Check sheet for the modelled part. Datum: model origin and axes. Units: mm. Face numbers are marked on the shaded views. A direction names the side the tool comes from. Give positions to 0.01 mm unless a question says otherwise; leave off trailing zeros. Loops run counter-clockwise (first coordinate to the right, second up) from the corner with the lowest first, then second, coordinate; pieces in that order, holes last. Notation, with made-up numbers: (83, -34.75) - (142, -34.75) arc R13 cw to (142, -16.75) - close; hole circle Ø7 at (80.25, 26). An arc over 180 degrees is marked (long way). Answer in a Markdown table with one row per item. Add a question column.
(1) Draft check along X on the marked faces 4, 5 and 6. Enter one of: released by +X, released by -X, zero draft, split by the parting line, or undercut.
(2) Set-up check for the marked faces 1, 2 and 3: record each of +Z, -Z, +X, -X, +Y, -Y from which the full face is reachable in a straight line by a thin tool's end or side.
(3) Thickness scan on L1, parallel to Z at x = -60, y = -1; L2, parallel to Z at x = -29, y = -3.5; L3, parallel to X at y = -0.5, z = -1.5. Record the ranges inside material, lowest first.
(4) Sectioned sample at C-C on y = -4.25. Enter the section's corners in (x, z) (1 decimal).
(5) Sectioned sample at D-D on x = -14. Enter the section's corners in (y, z), then the cut area to 3 significant figures.
(6) Sectioned sample at A-A on y = -11.5. Enter the section's corners in (x, z), then the cut area to 3 significant figures.
(7) Go/stop test with flat-tipped pins: P1, Ø13, axis at x = -14, z = 34.5, coming from the +Y side; P2, Ø1, axis at x = -86, z = 30, coming from the -Y side; P3, Ø4, axis at y = -6, z = 29, coming from the -X side. Record where each tip stops, or that it passes through.
(8) Sectioned sample at B-B on x = -56.5. Enter the section's corners in (y, z), then the cut area to 3 significant figures.
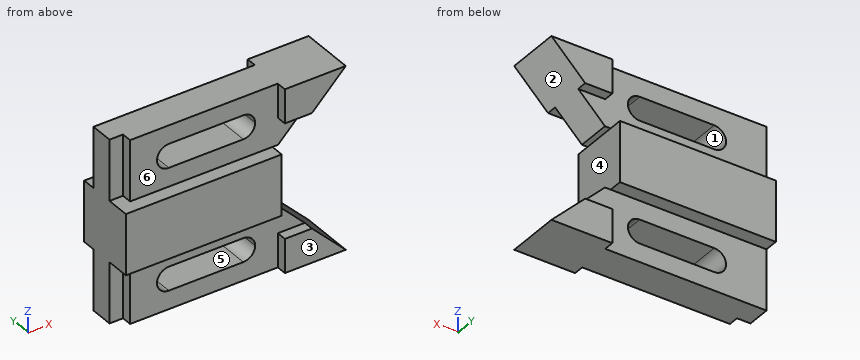
from build123d import *

# Parameters (mm, degrees)
F1_DEPTH = 104.648
F2_W     = 75.946
F2_H     = 4.826
F2_W_2   = 6.35
F3_DEPTH = 28.575
F5_DEPTH = 22.099
F7_DEPTH = 26.925
F9_DEPTH = 28.449


# Not quite as in the source:
# - a pattern or mirror of a feature is missing from the dataset's text; its kind, count and spacing are read off the source's solid


with BuildPart() as f1:
    # F0 (on Right) → F1 (new body)
    with BuildSketch(Plane.YZ):
        Polygon((7.874, -14.2875), (14.224, -14.2875), (14.224, 14.2875), (7.874, 14.2875), (-7.874, 14.2875), (-14.224, 14.2875), (-14.224, -14.2875), (-7.874, -14.2875), align=None)
        Polygon((-7.874, 14.2875), (7.874, 14.2875), (7.874, 26.924), (12.7, 26.924), (12.7, 42.8625), (0, 42.8625), (-12.7, 42.8625), (-12.7, 26.924), (-7.874, 26.924), align=None)
        Polygon((7.874, -26.924), (7.874, -14.2875), (-7.874, -14.2875), (-7.874, -26.924), (-12.7, -26.924), (-12.7, -42.8625), (0, -42.8625), (12.7, -42.8625), (12.7, -26.924), align=None)
    extrude(amount=-F1_DEPTH)

    # F2 (on face) → F3 (cut)
    with BuildSketch(Plane.XY.offset(42.8625)):
        Polygon((-98.298, -7.874), (-104.648, -7.874), (-104.648, -12.7), (-28.702, -12.7), (-28.702, -7.874), align=None)
        with Locations((-66.675, 10.287)):
            Rectangle(F2_W, F2_H)
        with Locations((-101.473, -5.461)):
            Rectangle(F2_W_2, F2_H)
    f3 = extrude(amount=-F3_DEPTH, mode=Mode.SUBTRACT)

    # F3_copies: F3 across plane
    add(f3.mirror(Plane(origin=(0, 0, 0), x_dir=(-1, 0, 0), z_dir=(0, 0, -1))), mode=Mode.SUBTRACT)

    # F4 (on face) → F5 (cut, through all)
    with BuildSketch(Plane.XZ.offset(7.874)):
        with BuildLine():
            ThreePointArc((-80.01, -34.2265), (-76.0586873067, -32.5898126933), (-74.422, -28.6385))
            ThreePointArc((-74.422, -28.6385), (-76.0586873067, -24.6871873067), (-80.01, -23.0505))
            ThreePointArc((-80.01, -23.0505), (-85.598, -28.6385), (-80.01, -34.2265))
        make_face()
        with BuildLine():
            ThreePointArc((-80.01, -23.0505), (-76.0586873067, -24.6871873067), (-74.422, -28.6385))
            ThreePointArc((-74.422, -28.6385), (-76.0586873067, -32.5898126933), (-80.01, -34.2265))
            Line((-80.01, -34.2265), (-44.958, -34.2265))
            ThreePointArc((-44.958, -34.2265), (-50.546, -28.6385), (-44.958, -23.0505))
            Line((-44.958, -23.0505), (-80.01, -23.0505))
        make_face()
        with BuildLine():
            ThreePointArc((-39.37, -28.6385), (-41.0066873067, -24.6871873067), (-44.958, -23.0505))
            ThreePointArc((-44.958, -23.0505), (-50.546, -28.6385), (-44.958, -34.2265))
            ThreePointArc((-44.958, -34.2265), (-41.0066873067, -32.5898126933), (-39.37, -28.6385))
        make_face()
    f5 = extrude(amount=-F5_DEPTH, mode=Mode.SUBTRACT)

    # F5_copies: F5 across plane
    add(f5.mirror(Plane.XY), mode=Mode.SUBTRACT)

    # F6 (on face) → F7 (cut, through all)
    with BuildSketch(Plane.XZ.offset(12.7)):
        Polygon((0, -14.2875), (-28.575, -14.2875), (0, -42.8625), align=None)
    f7 = extrude(amount=-F7_DEPTH, mode=Mode.SUBTRACT)

    # F7_copies: F7 across plane
    add(f7.mirror(Plane.XY), mode=Mode.SUBTRACT)

    # F8 (on face) → F9 (cut, through all)
    with BuildSketch(Plane.XZ.offset(14.224)):
        Polygon((-31.242, 14.2875), (-31.242, 0), (-31.242, -14.2875), (0, -14.2875), (0, 14.2875), align=None)
    extrude(amount=-F9_DEPTH, mode=Mode.SUBTRACT)


solid = f1.part
Reply:
| question | item | result |
|---|---|---|
| 1 | face 4 | released by +X |
| 1 | face 5 | undercut |
| 1 | face 6 | zero draft |
| 2 | face 1 | +Y, -Y |
| 2 | face 2 | +X, +Y, -Y |
| 2 | face 3 | +Z, -Z, +X, -X, -Y |
| 3 | L1 | -42.86 to -34.23, -23.05 to 23.05, 34.23 to 42.86 |
| 3 | L2 | -42.86 to -14.29, 14.29 to 42.86 |
| 3 | L3 | -104.65 to -31.24 |
| 4 | outline | (-104.6, -14.3) - (-98.3, -14.3) - (-98.3, -42.9) - (0, -42.9) - (-28.6, -14.3) - (-31.2, -14.3) - (-31.2, 14.3) - (-28.6, 14.3) - (0, 42.9) - (-98.3, 42.9) - (-98.3, 14.3) - (-104.6, 14.3) - close; hole (-80, -34.2) - (-45, -34.2) arc R5.6 ccw to (-45, -23.1) - (-80, -23.1) arc R5.6 ccw to start; hole (-80, 23.1) - (-45, 23.1) arc R5.6 ccw to (-45, 34.2) - (-80, 34.2) arc R5.6 ccw to start |
| 5 | outline | (-12.7, -42.86) - (12.7, -42.86) - (12.7, -28.86) - (-12.7, -28.86) - close; (-12.7, 28.86) - (12.7, 28.86) - (12.7, 42.86) - (-12.7, 42.86) - close |
| 5 | area | 711 mm^2 |
| 6 | outline | (-104.65, -14.29) - (-31.24, -14.29) - (-31.24, 14.29) - (-104.65, 14.29) - close; (-28.7, -42.86) - (0, -42.86) - (-15.94, -26.92) - (-28.7, -26.92) - close; (-28.7, 26.92) - (-15.94, 26.92) - (0, 42.86) - (-28.7, 42.86) - close |
| 6 | area | 2,760 mm^2 |
| 7 | P1 | y = 12.7 |
| 7 | P2 | y = -7.87 |
| 7 | P3 | x = -98.3 |
| 8 | outline | (-14.22, -14.29) - (-7.87, -14.29) - (-7.87, -23.05) - (7.87, -23.05) - (7.87, -14.29) - (14.22, -14.29) - (14.22, 14.29) - (7.87, 14.29) - (7.87, 23.05) - (-7.87, 23.05) - (-7.87, 14.29) - (-14.22, 14.29) - close; (-7.87, -42.86) - (7.87, -42.86) - (7.87, -34.23) - (-7.87, -34.23) - close; (-7.87, 34.23) - (7.87, 34.23) - (7.87, 42.86) - (-7.87, 42.86) - close |
| 8 | area | 1,360 mm^2 |
